Read the model definition and answer for the solid it produces. Units are mm, in the model's axes. A direction names the side the tool comes from. Round coordinates to 2 decimals unless told otherwise and drop trailing zeros. Loops run counter-clockwise (first coordinate to the right, second up) from the corner with the lowest first, then second, coordinate; pieces in that order, holes last. Notation, with made-up numbers: M -39,25.5 L -6,25.5 A23 cw -6,48.5 Z; hole C 89,71.5 d5. An arc over 180 degrees is marked long. Write each question's results on one line, items separated by ' | '.
```python
from build123d import *

# Parameters (mm, degrees)
BASE_EXTRUDE_DEPTH   = 12.7
MIRROR2_COPY_1_DEPTH = 12.7


with BuildPart() as part:
    # Sketch1 → Base-Extrude (new, symmetric)
    with BuildSketch(Plane.XY):
        with BuildLine():
            Line((0, 36.5125), (0, 2.6924))
            ThreePointArc((0, 2.6924), (0.788585702, 0.788585702), (2.6924, 0))
            Line((2.6924, 0), (38.5826, 0))
            ThreePointArc((38.5826, 0), (40.486414298, 0.788585702), (41.275, 2.6924))
            Line((41.275, 2.6924), (41.275, 36.5125))
            ThreePointArc((41.275, 36.5125), (36.5125, 41.275), (31.75, 36.5125))
            Line((31.75, 36.5125), (31.75, 35.47745))
            ThreePointArc((31.75, 35.47745), (33.0962, 34.13125), (34.4424, 35.47745))
            Line((34.4424, 35.47745), (34.4424, 36.5125))
            ThreePointArc((34.4424, 36.5125), (36.5125, 38.5826), (38.5826, 36.5125))
            Line((38.5826, 36.5125), (38.5826, 2.6924))
            Line((38.5826, 2.6924), (2.6924, 2.6924))
            Line((2.6924, 2.6924), (2.6924, 36.5125))
            ThreePointArc((2.6924, 36.5125), (4.7625, 38.5826), (6.8326, 36.5125))
            Line((6.8326, 36.5125), (6.8326, 35.47745))
            ThreePointArc((6.8326, 35.47745), (8.1788, 34.13125), (9.525, 35.47745))
            Line((9.525, 35.47745), (9.525, 36.5125))
            ThreePointArc((9.525, 36.5125), (4.7625, 41.275), (0, 36.5125))
        make_face()
    base_extrude = extrude(amount=BASE_EXTRUDE_DEPTH, both=True)

    # Mirror1: Base-Extrude across plane
    add(base_extrude.mirror(Plane(origin=(0, 0, 0), x_dir=(0, 0, 1), z_dir=(1, 0, 0))))

    # Mirror2: Base-Extrude across plane
    add(base_extrude.mirror(Plane.ZX))

    # Mirror2 copy 1 sketch → Mirror2 copy 1 (add, symmetric)
    with BuildSketch(Plane(origin=(0, 0, 0), x_dir=(-1, 0, 0), z_dir=(0, 0, 1))):
        with BuildLine():
            Line((0, 36.5125), (0, 2.6924))
            ThreePointArc((0, 2.6924), (0.788585702, 0.788585702), (2.6924, 0))
            Line((2.6924, 0), (38.5826, 0))
            ThreePointArc((38.5826, 0), (40.486414298, 0.788585702), (41.275, 2.6924))
            Line((41.275, 2.6924), (41.275, 36.5125))
            ThreePointArc((41.275, 36.5125), (36.5125, 41.275), (31.75, 36.5125))
            Line((31.75, 36.5125), (31.75, 35.47745))
            ThreePointArc((31.75, 35.47745), (33.0962, 34.13125), (34.4424, 35.47745))
            Line((34.4424, 35.47745), (34.4424, 36.5125))
            ThreePointArc((34.4424, 36.5125), (36.5125, 38.5826), (38.5826, 36.5125))
            Line((38.5826, 36.5125), (38.5826, 2.6924))
            Line((38.5826, 2.6924), (2.6924, 2.6924))
            Line((2.6924, 2.6924), (2.6924, 36.5125))
            ThreePointArc((2.6924, 36.5125), (4.7625, 38.5826), (6.8326, 36.5125))
            Line((6.8326, 36.5125), (6.8326, 35.47745))
            ThreePointArc((6.8326, 35.47745), (8.1788, 34.13125), (9.525, 35.47745))
            Line((9.525, 35.47745), (9.525, 36.5125))
            ThreePointArc((9.525, 36.5125), (4.7625, 41.275), (0, 36.5125))
        make_face()
    extrude(amount=MIRROR2_COPY_1_DEPTH, both=True)


solid = part.part
```
1. Find section B-B, the plane x = 5.5. Give the vertices of the cut face in (y, z).
Completed:
outline: M -41.22,-12.7 L -38.45,-12.7 L -38.45,12.7 L -41.22,12.7 Z; M -2.69,-12.7 L 2.69,-12.7 L 2.69,12.7 L -2.69,12.7 Z; M 38.45,-12.7 L 41.22,-12.7 L 41.22,12.7 L 38.45,12.7 Z
2. Given P1, Ø5, axis at x = -22, z = 5.5, coming from the +Y side; P2, Ø4, axis at x = -1, z = -4, coming from the +Y side; P3, Ø1, axis at x = 25.5, z = 8, coming from the -Y side, each flat-ended and moving along its own axis, determine where each tip first touches the part or whether it passes through.
Completed:
P1: stops at y = 2.69 | P2: stops at y = 40.94 | P3: stops at y = -2.69
3. Find section A-A, the plane y = -23. Give the vertices of the cut face in (x, z) (3 decimals), then the cut area to 3 significant figures.
Completed:
outline: M -41.275,-12.7 L -38.583,-12.7 L -38.583,12.7 L -41.275,12.7 Z; M -2.692,-12.7 L 2.692,-12.7 L 2.692,12.7 L -2.692,12.7 Z; M 38.583,-12.7 L 41.275,-12.7 L 41.275,12.7 L 38.583,12.7 Z | area: 274 mm2
4. Find section C-C, the plane x = 18. Give the vertices of the cut face in (y, z), then the cut area to 3 significant figures.
Completed:
outline: M -2.69,-12.7 L 2.69,-12.7 L 2.69,12.7 L -2.69,12.7 Z | area: 137 mm2
5. Find the intervals of material crossed by L1, parallel to X at y = -20, z = 3.5 (3 decimals); L2, parallel to Y at x = -3, z = -10; L3, parallel to Y at x = 33, z = -10, in increasing order.
Completed:
L1: x = -41.275 to -38.583, -2.692 to 2.692, 38.583 to 41.275 | L2: y = -40.94 to -37.6, -2.69 to 2.69, 37.6 to 40.94 | L3: y = -39.73 to -34.13, -2.69 to 2.69, 34.13 to 39.73
6. Which of the six approach directions +Z, -Z, +X, -X, +Y, -Y give full straight-line access (tool end or side, diameter ignored) to faces 1 (the face through (-41.275, -19, 0)), 2 (the face through (-33.07, 34.13, 0.18))?
Completed:
face 1: +Z, -Z, -X, +Y, -Y | face 2: +Z, -Z
